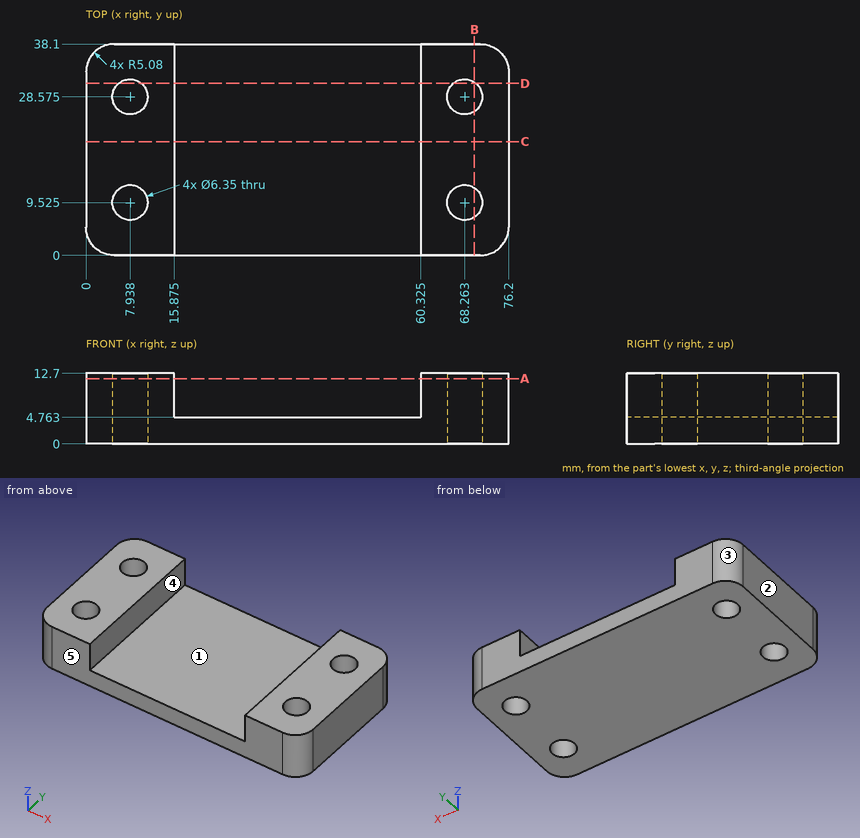
Can you work these out from the drawing? Everything is in mm from the part's minimum corner. A direction names the side the tool comes from. Coordinates: 2 decimals unless noted, no trailing zeros. Order: outer loops, then holes, each group sorted by start corner. A loop starts at its lowest first (then second) coordinate and runs counter-clockwise, first axis right, second up. Notation, with made-up numbers: M 35.25,62 L 69.25,62 A22 ccw 69.25,87 Z; hole C 27,-31.75 d10. An arc over 180 degrees is marked long. Answer as CSV lines item,"result". Start each with the question number.
1. I want a section at A-A, the plane z = 11.75. Count the separate pieces of the cut face and the enclosed holes in it, and give its area (3 significant figures).
2. I want a section at D-D, the plane y = 31. Write out the boundary of the cut face in (x, z) (1 decimal).
3. I need wall thicknesses on line 1 (Y direction, x = 68.5, z = 9.5); line 2 (X direction, y = 32.5, z = 5) (1 decimal); line 3 (Y direction, x = 70.5, z = 2.5) (1 decimal). Which ranges of each line are inside material? Lowest first, please. Write a range as [from, to].
4. For pin 1 (1.5 mm diameter, centred on x = 30, z = 6.5, fed in from -Y); pin 2 (11.5 mm diameter, centred on x = 28, y = 12.5, fed in from +Z), each with a flat end and sliding along its axis, tell me the tip position at first contact or that it passes through.
5. On a 3-axis mill with a long thin cutter (end or side, diameter ignored), from which of +Z, -Z, +X, -X, +Y, -Y can I reach the whole of each face in a straight line? I mean the marked faces 1 and 2. Say none if no direction works.
6. We'd pull the mould along X, two halves only. Please class the marked faces 3, 4 and 5: released by +X, released by -X, zero draft, split by the parting line, or undercut.
7. I want a section at C-C, the plane y = 20.5. Write out the boundary of the cut face in (x, z) (1 decimal).
8. I want a section at B-B, the plane x = 70. Write out the boundary of the cut face in (y, z), and give its area (3 significant figures).
Recorded:
1,separate pieces,"2"
1,enclosed holes,"4"
1,area,"1,060 mm2"
2,outline,"M 0,0 L 5.9,0 L 5.9,12.7 L 0,12.7 Z; M 10,0 L 66.2,0 L 66.2,12.7 L 60.3,12.7 L 60.3,4.8 L 15.9,4.8 L 15.9,12.7 L 10,12.7 Z; M 70.3,0 L 76.2,0 L 76.2,12.7 L 70.3,12.7 Z"
3,line 1,"y = [0, 6.36], [12.69, 25.41], [31.74, 38.1]"
3,line 2,"x = [0, 15.9], [60.3, 76.2]"
3,line 3,"y = [0, 7.3], [11.8, 26.3], [30.8, 38.1]"
4,pin 1,"passes through"
4,pin 2,"stops at z = 4.76"
5,face 1,"+Z, +Y, -Y"
5,face 2,"+Z, -Z, -X, +Y, -Y"
6,face 3,"released by -X"
6,face 4,"undercut"
6,face 5,"zero draft"
7,outline,"M 0,0 L 76.2,0 L 76.2,12.7 L 60.3,12.7 L 60.3,4.8 L 15.9,4.8 L 15.9,12.7 L 0,12.7 Z"
8,outline,"M 0,0 L 6.87,0 L 6.87,12.7 L 0,12.7 Z; M 12.18,0 L 25.92,0 L 25.92,12.7 L 12.18,12.7 Z; M 31.23,0 L 38.1,0 L 38.1,12.7 L 31.23,12.7 Z"
8,area,"349 mm2"
